```python
from build123d import *

# Parameters (mm, degrees)
SKETCH1_W               = 9
SKETCH1_H               = 10
SKETCH1_W_2             = 5
SKETCH1_H_2             = 6
BOSS_EXTRUDE1_DEPTH     = 15
BOSS_EXTRUDE2_DEPTH     = 2
SKETCH3_R               = 0.95
CUT_EXTRUDE2_DEPTH      = 1
CUT_EXTRUDE2_DEPTH_BACK = 10
SKETCH5_R               = 1.5
SKETCH5_R_2             = 0.95
BOSS_EXTRUDE3_DEPTH     = 5
SKETCH6_R               = 0.5
CUT_EXTRUDE3_DEPTH      = 11
SKETCH7_W               = 0.25
SKETCH7_H               = 25.68334021
SKETCH7_H_2             = 27.406815516
CUT_EXTRUDE4_DEPTH      = 1
CUT_EXTRUDE4_DEPTH_BACK = 11
SKETCH8_R               = 2.5
SKETCH8_R_2             = 1.5
BOSS_EXTRUDE4_DEPTH     = 2


with BuildPart() as part:
    # Sketch1 → Boss-Extrude1 (new body)
    with BuildSketch(Plane(origin=(0, 0, 0), x_dir=(1, 0, 0), z_dir=(0, 1, 0))):
        Rectangle(SKETCH1_W, SKETCH1_H)
        Rectangle(SKETCH1_W_2, SKETCH1_H_2, mode=Mode.SUBTRACT)
    extrude(amount=BOSS_EXTRUDE1_DEPTH)

    # Sketch2 → Boss-Extrude2 (add)
    with BuildSketch(Plane(origin=(4.5, 0, 0), x_dir=(0, 0, -1), z_dir=(1, 0, 0))):
        with BuildLine():
            Line((5, -10), (5, 0))
            Line((5, 0), (-5, 0))
            ThreePointArc((-5, 0), (-2.071067812, -7.071067812), (5, -10))
        make_face()
    boss_extrude2 = extrude(amount=-BOSS_EXTRUDE2_DEPTH)

    # Mirror1: Boss-Extrude2 across plane
    add(boss_extrude2.mirror(Plane(origin=(0, 0, 0), x_dir=(0, 0, 1), z_dir=(1, 0, 0))))

    # Sketch3 → Cut-Extrude2 (cut, two sides)
    with BuildSketch(Plane(origin=(4.5, 0, 0), x_dir=(0, 0, -1), z_dir=(1, 0, 0))) as cut_extrude2_sk:
        with Locations((0, -5)):
            Circle(SKETCH3_R)
    extrude(amount=CUT_EXTRUDE2_DEPTH, mode=Mode.SUBTRACT)
    extrude(cut_extrude2_sk.sketch, amount=-CUT_EXTRUDE2_DEPTH_BACK, mode=Mode.SUBTRACT)

    # Sketch5 → Boss-Extrude3 (add)
    with BuildSketch(Plane(origin=(-2.5, 0, 0), x_dir=(0, 0, -1), z_dir=(1, 0, 0))):
        with Locations((0, -5)):
            Circle(SKETCH5_R)
        with Locations((0, -5)):
            Circle(SKETCH5_R_2, mode=Mode.SUBTRACT)
    extrude(amount=BOSS_EXTRUDE3_DEPTH)

    # Sketch6 → Cut-Extrude3 (cut, through all)
    with BuildSketch(Plane.XY.offset(5)):
        with Locations((0, 3)):
            Circle(SKETCH6_R)
        with Locations((0, 6)):
            Circle(SKETCH6_R)
    extrude(amount=-CUT_EXTRUDE3_DEPTH, mode=Mode.SUBTRACT)

    # Sketch7 → Cut-Extrude4 (cut, two sides)
    with BuildSketch(Plane.XY.offset(5)) as cut_extrude4_sk:
        with Locations((-4.375, 2.158329895)):
            Rectangle(SKETCH7_W, SKETCH7_H)
        with Locations((4.375, 1.296592242)):
            Rectangle(SKETCH7_W, SKETCH7_H_2)
    extrude(amount=CUT_EXTRUDE4_DEPTH, mode=Mode.SUBTRACT)
    extrude(cut_extrude4_sk.sketch, amount=-CUT_EXTRUDE4_DEPTH_BACK, mode=Mode.SUBTRACT)

    # Sketch8 → Boss-Extrude4 (add)
    with BuildSketch(Plane.ZY.offset(-2.5)):
        with Locations((0, -5)):
            Circle(SKETCH8_R)
        with Locations((0, -5)):
            Circle(SKETCH8_R_2, mode=Mode.SUBTRACT)
    boss_extrude4 = extrude(amount=BOSS_EXTRUDE4_DEPTH)

    # Mirror2: Boss-Extrude4 across plane
    add(boss_extrude4.mirror(Plane(origin=(0, 0, 0), x_dir=(0, 0, 1), z_dir=(1, 0, 0))))


solid = part.part
```
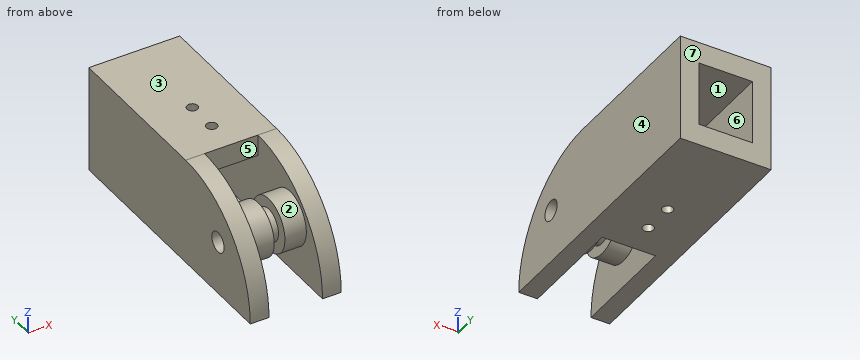
Read the model definition and answer for the solid it produces. Units are mm, in the model's axes. Face numbers are marked on the shaded views. A direction names the side the tool comes from. Coordinates: 2 decimals unless noted, no trailing zeros. Write each loop counter-clockwise with the first axis right and the second up, starting at its lowest first coordinate (ties: lowest second). Pieces come first, ordered by that corner, then holes. Notation, with made-up numbers: (69, -3) - (98, -3) arc R24 ccw to (98, 7) - close; hole circle Ø5 at (11.25, -19.75). An arc over 180 degrees is marked (long way). Answer as a JSON object with one key per item and string values. Group by question number.
1. A cutting plane is placed at C-C (x = 0). Determine the outline of the cut face in (y, z), plus the area to 3 significant figures.
2. A cutting plane is placed at B-B (y = 3). Determine the outline of the cut face in (x, z), plus the area to 3 significant figures.
3. Which of the six approach directions +Z, -Z, +X, -X, +Y, -Y give full straight-line access (tool end or side, diameter ignored) to the marked faces 5, 6 and 7?
4. Consider L1, parallel to Y at x = 0, z = 3.45; L2, parallel to X at y = 12, z = -2.5; L3, parallel to Z at x = -0.5, y = 13.5. Determine where each line is inside the solid, lowest interval first. Write a range as [from, to].
5. A cutting plane is placed at A-A (x = 2). Determine the outline of the cut face in (y, z), plus the area to 3 significant figures.
6. A cutting plane is placed at D-D (z = -2). Determine the outline of the cut face in (x, y).
7. The mould has two halves that part along X. Classify the marked faces 1, 2, 3 and 4: +X half, -X half, draft (parallel to the pull), parting line (faces both ways), or undercut.
8. Each of these flat-tipped pins is pushed along its axis until it touches: P1, Ø2, axis at x = 0.5, z = -4, coming from the -Y side; P2, Ø3, axis at x = -3, z = -1.5, coming from the -Y side. Where does it stop, or does it pass through?
Worked out:
{
 "1": {"outline": "circle Ø3 at (-5, 0); (0, -5) - (2.5, -5) - (2.5, -3) - (0, -3) - close; (0, 3) - (2.5, 3) - (2.5, 5) - (0, 5) - close; (3.5, -5) - (5.5, -5) - (5.5, -3) - (3.5, -3) - close; (3.5, 3) - (5.5, 3) - (5.5, 5) - (3.5, 5) - close; (6.5, -5) - (15, -5) - (15, -3) - (6.5, -3) - close; (6.5, 3) - (15, 3) - (15, 5) - (6.5, 5) - close; hole circle Ø1.9 at (-5, 0)", "area": "56.2 mm²"},
 "2": {"outline": "(-4.25, -5) - (-0.5, -5) - (-0.5, -3) - (-2.5, -3) - (-2.5, 3) - (-0.5, 3) - (-0.5, 5) - (-4.25, 5) - close; (0.5, -5) - (4.25, -5) - (4.25, 5) - (0.5, 5) - (0.5, 3) - (2.5, 3) - (2.5, -3) - (0.5, -3) - close", "area": "51.0 mm²"},
 "3": {"face 5": "+Z, -Z, -Y", "face 6": "none", "face 7": "+Z, -Z, +X, -X, +Y"},
 "4": {"L1": "y = [0, 2.5], [3.5, 5.5], [6.5, 15]", "L2": "x = [-4.25, -2.5], [2.5, 4.25]", "L3": "z = [-5, -3], [3, 5]"},
 "5": {"outline": "circle Ø5 at (-5, 0); (0, -5) - (15, -5) - (15, -3) - (0, -3) - close; (0, 3) - (15, 3) - (15, 5) - (0, 5) - close; hole circle Ø1.9 at (-5, 0)", "area": "76.8 mm²"},
 "6": {"outline": "(-4.25, -9.54) - (-2.5, -9.54) - (-2.5, -6.5) - (-0.5, -6.5) - (-0.5, -3.5) - (-2.5, -3.5) - (-2.5, 15) - (-4.25, 15) - close; (0.5, -6.5) - (2.5, -6.5) - (2.5, -9.54) - (4.25, -9.54) - (4.25, 15) - (2.5, 15) - (2.5, -3.5) - (0.5, -3.5) - close"},
 "7": {"face 1": "undercut", "face 2": "undercut", "face 3": "draft", "face 4": "+X half"},
 "8": {"P1": "stops at y = 0", "P2": "stops at y = -9.8"}
}
